```python
from build123d import *

# Parameters (mm, degrees)
F1_DEPTH = 152.4
F3_D     = 3.81
F5_D     = 3.81


with BuildPart() as f1:
    # F0 (on Front) → F1 (new body, symmetric)
    with BuildSketch(Plane.XZ):
        Polygon((12.7, 25.4), (-12.7, 25.4), (-12.7, -25.4), (12.7, -25.4), (12.7, -22.225), (-9.525, -22.225), (-9.525, 22.225), (12.7, 22.225), align=None)
    extrude(amount=F1_DEPTH, both=True)

    # F3 (through all)
    with Locations(Plane(origin=(0, 0, -25.4), x_dir=(1, 0, 0), z_dir=(0, 0, -1))):
        with Locations((6.35, -136.525), (5.915893, -60.325), (6.35, 34.925), (6.35, 111.125)):
            Hole(F3_D / 2)

    # F5 (through all)
    with Locations(Plane(origin=(-12.7, 0, 0), x_dir=(0, -1, 0), z_dir=(-1, 0, 0))):
        with Locations((117.475, -12.7), (117.475, 12.7), (-142.875, -12.7), (-142.875, 12.7)):
            Hole(F5_D / 2)


solid = f1.part
```
Part model, mm, in its own coordinate system. A direction names the side the tool comes from. Give positions to 0.01 mm unless a question says otherwise; leave off trailing zeros. Write each loop counter-clockwise with the first axis right and the second up, starting at its lowest first coordinate (ties: lowest second). Pieces come first, ordered by that corner, then holes. Notation, with made-up numbers: (30, 17.5) -> (60, 17.5) arc R26 cw to (60, 44.5) -> close; hole circle Ø3 at (38.25, 56.25). An arc over 180 degrees is marked (long way). Put each result on its own line as item: value. Start each with the question number.
Item 1: Wall check: L1, parallel to Y at x = 6.35, z = 23; L2, parallel to Z at x = -1.75, y = -53.5 (3 decimals); L3, parallel to X at y = 10.5, z = -9 (3 decimals). Give the ranges that are in metal, low to high. Write a range as [from, to].
Item 2: Pull direction Z, two halves, no side cores. Call faces 1 (the face through (0, -2, -25.4)), 2 (the face through (-12.7, -2, 0)), 3 (the face through (-9.525, -2, 0)): pulls with the +Z half, pulls with the -Z half, needs draft (parallel to the pull), parting line crosses it, or undercut.
Item 3: Cut at A-A (x = -2.5). List the corners of the cut face in (y, z) (3 decimals).
Item 4: Cut at B-B (y = 31.5). List the corners of the cut face in (x, z) (3 decimals), then the cut area to 3 significant figures.
Item 5: Which spindle directions (+Z, -Z, +X, -X, +Y, -Y) get a long thin tool onto all of the face, cutting with end or side? Do faces 4 (the face through (1, -2, 22.225)), 5 (the face through (0, -2, 25.4)). Say none if no direction does.
Item 6: Cut at C-C (z = -1.5). List the corners of the cut face in (x, y) (3 decimals), then the cut area to 3 significant figures.
Item 7: Pin check, flat tips, straight feed: pin 1 Ø6 at (x, y) = (5.92, 60.32) entering from -Z; pin 2 Ø8 at (y, z) = (-112.5, 1.5) entering from +X (3 decimals); pin 3 Ø12 at (x, z) = (0, 0) entering from +Y. Stop position of each tip, or through.
Answer list:
1. L1: y = [-152.4, -113.03], [-109.22, -36.83], [-33.02, 58.47], [62.18, 134.62], [138.43, 152.4]
1. L2: z = [-25.4, -22.225], [22.225, 25.4]
1. L3: x = [-12.7, -9.525]
2. face 1: pulls with the -Z half
2. face 2: needs draft
2. face 3: undercut
3. outline: (-152.4, -25.4) -> (152.4, -25.4) -> (152.4, -22.225) -> (-152.4, -22.225) -> close; (-152.4, 22.225) -> (152.4, 22.225) -> (152.4, 25.4) -> (-152.4, 25.4) -> close
4. outline: (-12.7, -25.4) -> (12.7, -25.4) -> (12.7, -22.225) -> (-9.525, -22.225) -> (-9.525, 22.225) -> (12.7, 22.225) -> (12.7, 25.4) -> (-12.7, 25.4) -> close
4. area: 302 mm2
5. face 4: +X, +Y, -Y
5. face 5: +Z, +X, -X, +Y, -Y
6. outline: (-12.7, -152.4) -> (-9.525, -152.4) -> (-9.525, 152.4) -> (-12.7, 152.4) -> close
6. area: 968 mm2
7. pin 1: stops at z = -25.4
7. pin 2: stops at x = -9.525
7. pin 3: passes through
